Geometry: see drawing. Coordinates: mm, zero at the bounding-box minimum. Round coordinates to 2 decimals unless told otherwise and drop trailing zeros. Write each loop counter-clockwise with the first axis right and the second up, starting at its lowest first coordinate (ties: lowest second). Pieces come first, ordered by that corner, then holes. Notation, with made-up numbers: M 15.5,49.25 L 48.5,49.25 A20 cw 48.5,55.25 Z; hole C 12.25,-4 d8. An arc over 180 degrees is marked long. Use a Markdown table: item, result.
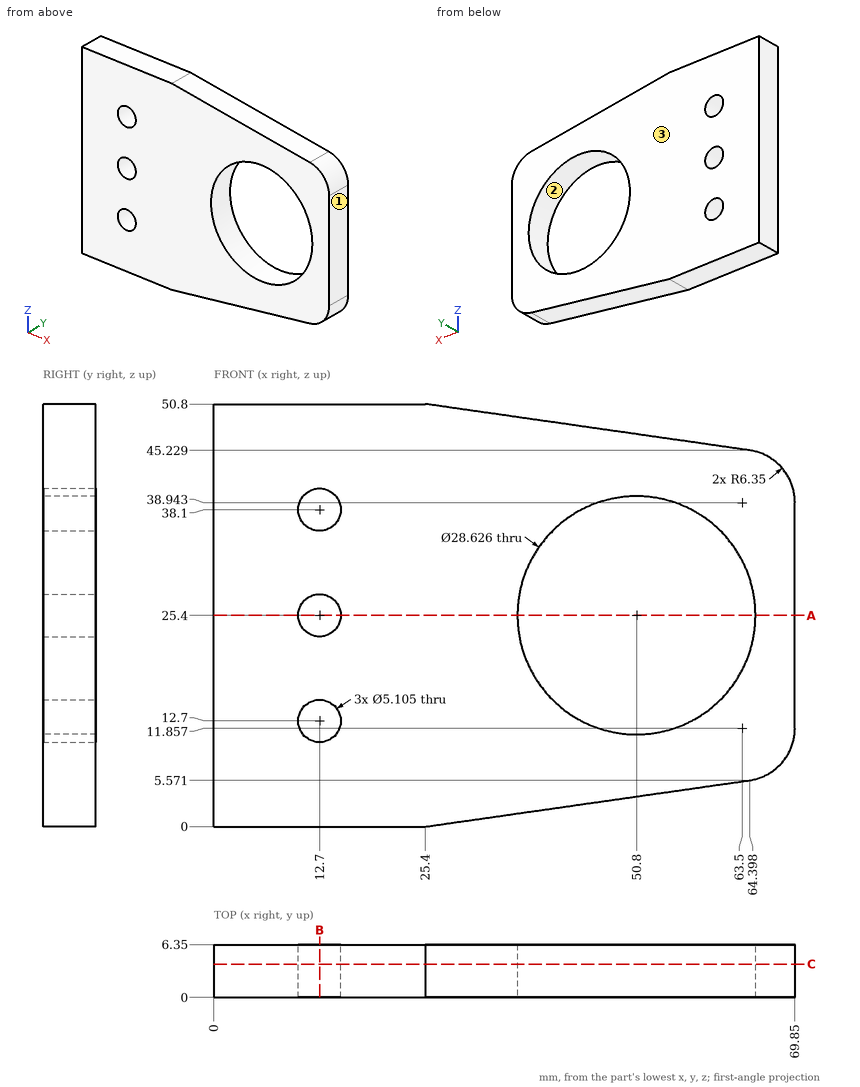
Q1. Section B-B on x = 12.7. Return loops of the section in (y, z), plus the area to 3 significant figures.
Results are:
| item | result |
|---|---|
| outline | M 0,0 L 6.35,0 L 6.35,10.15 L 0,10.15 Z; M 0,15.25 L 6.35,15.25 L 6.35,22.85 L 0,22.85 Z; M 0,27.95 L 6.35,27.95 L 6.35,35.55 L 0,35.55 Z; M 0,40.65 L 6.35,40.65 L 6.35,50.8 L 0,50.8 Z |
| area | 225 mm^2 |
Q2. Section A-A on z = 25.4. Return loops of the section in (x, y), plus the area to 3 significant figures.
Results are:
| item | result |
|---|---|
| outline | M 0,0 L 10.15,0 L 10.15,6.35 L 0,6.35 Z; M 15.25,0 L 36.49,0 L 36.49,6.35 L 15.25,6.35 Z; M 65.11,0 L 69.85,0 L 69.85,6.35 L 65.11,6.35 Z |
| area | 229 mm^2 |
Q3. Section C-C on y = 4. Give the number of separate pieces and of enclosed holes in the cut face, plus the area to 3 significant figures.
Results are:
| item | result |
|---|---|
| separate pieces | 1 |
| enclosed holes | 4 |
| area | 2,550 mm^2 |
Q4. Line query: L1, parallel to Z at x = 12.7, y = 4.5; L2, parallel to Z at x = 57, y = 1.75 (1 decimal); L3, parallel to Z at x = 44.5, y = 4.75. Output: solid intervals per line, ascending.
Results are:
| item | result |
|---|---|
| L1 | 0 to 10.15, 15.25 to 22.85, 27.95 to 35.55, 40.65 to 50.8 |
| L2 | 4.5 to 12.5, 38.3 to 46.3 |
| L3 | 2.73 to 12.55, 38.25 to 48.07 |
Q5. Mould query, pull axis X, two halves, no side actions, for the marked faces 1, 2 and 3. Classes: +X half, -X half, draft (parallel to the pull), parting line (faces both ways), or undercut.
Results are:
| item | result |
|---|---|
| face 1 | +X half |
| face 2 | undercut |
| face 3 | draft |
Q6. First-contact query: pin 1 Ø4.5 at (x, z) = (12.7, 12.7) entering from -Y; pin 2 Ø1.5 at (x, y) = (56.5, 2.5) entering from -Z. Flat tips, straight axial feed; report the tip coordinate or a pass-through.
Results are:
| item | result |
|---|---|
| pin 1 | through |
| pin 2 | z = 4.34 |
